Geometry check sheet. Reference: drawing and pictorial views, mm from the part's lowest x, y, z. Coordinates: 2 decimals unless noted, no trailing zeros. Write each loop counter-clockwise with the first axis right and the second up, starting at its lowest first coordinate (ties: lowest second). Pieces come first, ordered by that corner, then holes. Notation, with made-up numbers: (-30.75, 14.25) - (18.25, 14.25) arc R17 cw to (18.25, 39.25) - close; hole circle Ø7 at (52.5, -33.75). An arc over 180 degrees is marked (long way). Use one line per item in the form item = value. Start each with the question number.
(1) Mould release check, pull along X, two halves, no side actions. Record for the marked faces 1, 2 and 3: released by +X, released by -X, zero draft, split by the parting line, or undercut.
(2) Sectioned sample at D-D (y = 34.5). Record the cut outline in (x, z).
(3) Gauge pin test, flat ends, axial feed: pin 1 Ø6 at (x, z) = (40, 46.5) entering from -Y; pin 2 Ø4 at (x, y) = (26.5, 1.5) entering from +Z; pin 3 Ø0.9 at (x, y) = (11.5, 2.5) entering from +Z. Record the tip position at first contact, or that the pin passes through.
(4) Sectioned sample at A-A (y = 15.5). Record the cut outline in (x, z).
(5) Sectioned sample at C-C (z = 30). Record the cut outline in (x, y), and give its area (3 significant figures).
(6) Sectioned sample at B-B (x = 56). Record the cut outline in (y, z), and give its area (3 significant figures).
(7) Material ranges on line 1 (X direction, y = 26.5, z = 31.5); line 2 (X direction, y = 19.5, z = 61.5); line 3 (Y direction, x = 46, z = 56), recorded low to high. Write a range as [from, to].
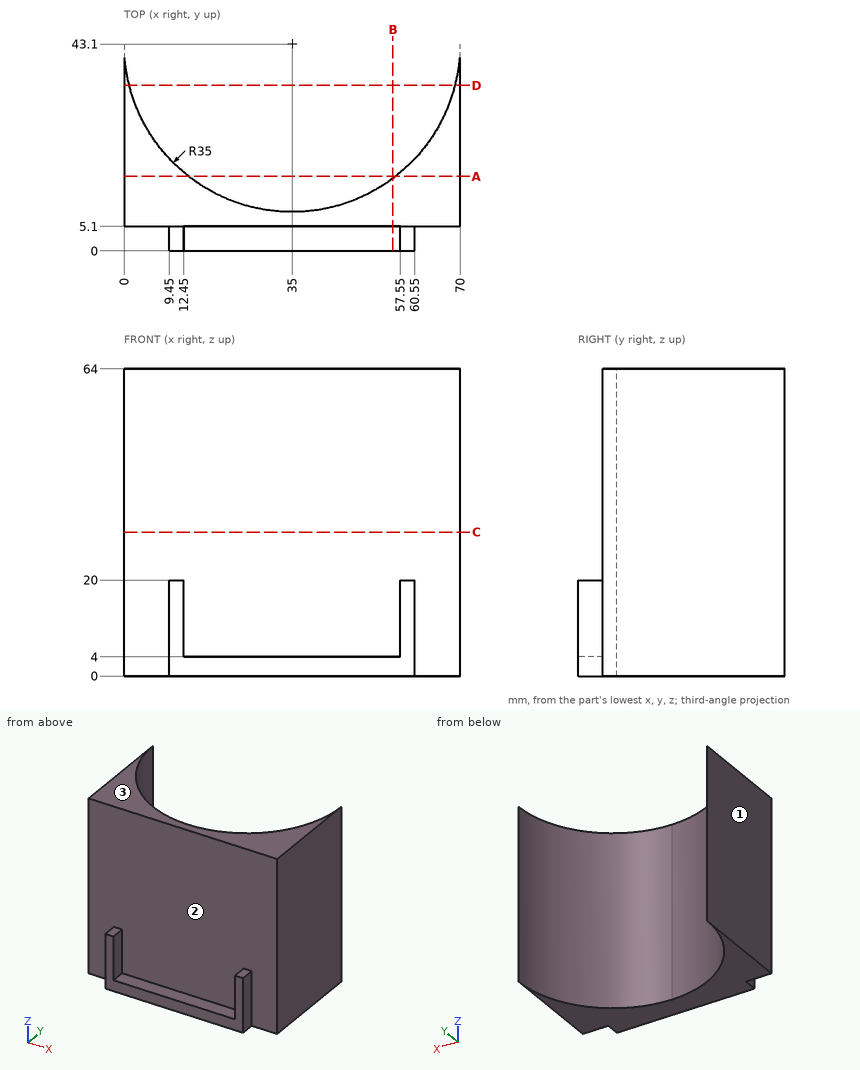
Answers below:
q1.face_1 = released by -X
q1.face_2 = undercut
q1.face_3 = zero draft
q2.outline = (0, 0) - (1.07, 0) - (1.07, 64) - (0, 64) - close; (68.93, 0) - (70, 0) - (70, 64) - (68.93, 64) - close
q3.pin_1 = 5.1
q3.pin_2 = 4
q3.pin_3 = 20
q4.outline = (0, 0) - (13.48, 0) - (13.48, 64) - (0, 64) - close; (56.52, 0) - (70, 0) - (70, 64) - (56.52, 64) - close
q5.outline = (0, 5.1) - (70, 5.1) - (70, 43.1) arc R35 cw to (35, 8.1) arc R35 cw to (0, 43.1) - close
q5.area = 736 mm2
q6.outline = (0, 0) - (15.1, 0) - (15.1, 64) - (5.1, 64) - (5.1, 4) - (0, 4) - close
q6.area = 660 mm2
q7.line_1 = [0, 4.19], [65.81, 70]
q7.line_2 = [0, 9.15], [60.85, 70]
q7.line_3 = [5.1, 9.87]
